from build123d import *

# Parameters (mm, degrees)
SKETCH1_R           = 25
SKETCH1_R_2         = 6
BOSS_EXTRUDE1_DEPTH = 16.5
CUT_EXTRUDE3_DEPTH  = 30


with BuildPart() as part:
    # Sketch1 → Boss-Extrude1 (new body)
    with BuildSketch(Plane(origin=(0, 0, 0), x_dir=(0, 0, -1), z_dir=(1, 0, 0))):
        Circle(SKETCH1_R)
        Circle(SKETCH1_R_2, mode=Mode.SUBTRACT)
    extrude(amount=BOSS_EXTRUDE1_DEPTH)

    # Sketch4 → Cut-Extrude3 (cut)
    with BuildSketch(Plane(origin=(16.5, 0, 0), x_dir=(0, 0, -1), z_dir=(1, 0, 0))):
        with BuildLine():
            Line((-16.75, 8.25), (-27.17881333, 8.25))
            Line((-27.17881333, 8.25), (-27.17881333, -8.25))
            Line((-27.17881333, -8.25), (-16.75, -8.25))
            ThreePointArc((-16.75, -8.25), (-8.5, 0), (-16.75, 8.25))
        make_face()
        with BuildLine():
            Line((2.670181604, 18.479586852), (-0.552498946, 28.397977726))
            Line((-0.552498946, 28.397977726), (-16.244931465, 23.299197319))
            Line((-16.244931465, 23.299197319), (-13.022250915, 13.380806444))
            ThreePointArc((-13.022250915, 13.380806444), (-2.626644452, 8.083980389), (2.670181604, 18.479586852))
        make_face()
        with BuildLine():
            Line((18.400262987, 3.171012772), (26.837350202, 9.300915446))
            Line((26.837350202, 9.300915446), (17.138893539, 22.649695854))
            Line((17.138893539, 22.649695854), (8.701806324, 16.519793179))
            ThreePointArc((8.701806324, 16.519793179), (6.876644452, 4.996174644), (18.400262987, 3.171012772))
        make_face()
        with BuildLine():
            Line((8.701806324, -16.519793179), (17.138893539, -22.649695854))
            Line((17.138893539, -22.649695854), (26.837350202, -9.300915446))
            Line((26.837350202, -9.300915446), (18.400262987, -3.171012772))
            ThreePointArc((18.400262987, -3.171012772), (6.876644452, -4.996174644), (8.701806324, -16.519793179))
        make_face()
        with BuildLine():
            Line((-13.022250915, -13.380806444), (-16.244931465, -23.299197319))
            Line((-16.244931465, -23.299197319), (-0.552498946, -28.397977726))
            Line((-0.552498946, -28.397977726), (2.670181604, -18.479586852))
            ThreePointArc((2.670181604, -18.479586852), (-2.626644452, -8.083980389), (-13.022250915, -13.380806444))
        make_face()
    extrude(amount=-CUT_EXTRUDE3_DEPTH, mode=Mode.SUBTRACT)

    # Sketch6 → Revolve1 (revolve)
    with BuildSketch(Plane(origin=(0, 0, 0), x_dir=(1, 0, 0), z_dir=(0, 1, 0))):
        Polygon((0, -25), (16.5, -8.5), (0, -8.5), align=None)
    revolve(axis=Axis((27.230838135, 0, 0), (-1, 0, 0)))


solid = part.part
Design review of the part built by this model. Coordinates are the model's own, in mm. A direction names the side the tool comes from. Round coordinates to 2 decimals unless told otherwise and drop trailing zeros. Loops run counter-clockwise (first coordinate to the right, second up) from the corner with the lowest first, then second, coordinate; pieces in that order, holes last. Notation, with made-up numbers: (21.5, 66) - (76.5, 66) arc R34 ccw to (76.5, 104) - close; hole circle Ø9 at (5.25, 60.25). An arc over 180 degrees is marked (long way). One line per item, written item: value. Start each with the question number.
1) Insertion check: pin 1 Ø2 at (x, z) = (5.5, 19) entering from -Y; pin 2 Ø1.5 at (x, z) = (10, -18.5) entering from +Y; pin 3 Ø3 at (x, z) = (15, -6) entering from -Y. Each pin has a flat end and moves straight along its axis. Give the tip position at first contact, or say it passes through.
2) To check wall thickness, follow L1, parallel to Y at x = 11.75, z = -11.5; L2, parallel to Z at x = 16, y = 4.5; L3, parallel to Z at x = 8, y = -4. State the ranges of each line that lie inside material, in increasing order. Write a range as from..to.
3) Consider section B-B on x = 1. Give the boundary of the cut face in (y, z), then the cut area to 3 significant figures.
4) For faces 1 (the cylindrical face through (12.616, -7.515, 13.346)), 2 (the cylindrical face through (12.616, -1.765, -15.214)), 3 (the flat face through (10.2, -18.5, -11.43)), 4 (the flat face through (10.2, 16.7, 14.1)), list the 3-axis set-ups (+Z, -Z, +X, -X, +Y, -Y) from which the entire face can be reached by the end or side of a thin tool; tool diameter is ignored.
Reported:
1. pin 1: stops at y = -17.35
1. pin 2: stops at y = 3.79
1. pin 3: stops at y = -24.59
2. L1: y = -22.2..-18.55, -6.58..6.58, 18.55..22.2
2. L2: z = -24.59..-20.23, -7.79..-3.97, 3.97..9.84
2. L3: z = -24.68..-19.54, -16.52..-4.47, 4.47..16.52
3. outline: (-24.99, -0.55) arc R25 ccw to (-20.55, -14.24) - (-19.92, -13.38) arc R24 ccw to (-6.57, -23.08) - (-7.2, -23.94) arc R25 ccw to (7.2, -23.94) - (6.57, -23.08) arc R24 ccw to (19.92, -13.38) - (20.55, -14.24) arc R25 ccw to (24.99, -0.55) - (23.98, -0.88) arc R24 ccw to (18.89, 14.81) - (19.9, 15.14) arc R25 ccw to (8.25, 23.6) - (8.25, 22.54) arc R24 ccw to (-8.25, 22.54) - (-8.25, 23.6) arc R25 ccw to (-19.9, 15.14) - (-18.89, 14.81) arc R24 ccw to (-23.98, -0.88) - close; hole circle Ø12 at (0, 0)
3. area: 1,770 mm^2
4. face 1: +Z, +X
4. face 2: +X
4. face 3: -Z, +X
4. face 4: +X, +Y
